Check sheet for the drawn part. Datum: minimum x, y, z corner. Units: mm. A direction names the side the tool comes from. Coordinates: 2 decimals unless noted, no trailing zeros. Write each loop counter-clockwise with the first axis right and the second up, starting at its lowest first coordinate (ties: lowest second). Pieces come first, ordered by that corner, then holes. Notation, with made-up numbers: M 69,-35.5 L 127,-35.5 A16 cw 127,-28.5 Z; hole C 67.5,0.5 d4. An arc over 180 degrees is marked long. Answer as CSV lines item,"result". Start each with the question number.
Q1. Mould release check, pull along X, two halves, no side actions. Record for the marked faces 1, 2, 3 and 4: pulls with the +X half, pulls with the -X half, needs draft (parallel to the pull), parting line crosses it, or undercut.
Q2. Thickness scan on line 1 along X through (y, z) = (13.5, 0.8); line 2 along Y through (x, z) = (22.5, 2.15). Record the ranges inside material, lowest first. Write a range as from..to.
Q3. Sectioned sample at A-A, the plane x = 13.5. Record the cut outline in (y, z).
Q4. Depth check by flat-ended pin: pin 1 Ø1.5 at (y, z) = (7.5, 2) entering from -X; pin 2 Ø1.5 at (x, z) = (6, 2) entering from -Y; pin 3 Ø1.5 at (x, z) = (21, 1.5) entering from +Y; pin 4 Ø3.5 at (x, y) = (22.5, 13.5) entering from -Z. Enter the tip coordinate at first touch or a pass-through.
Q5. Sectioned sample at D-D, the plane y = 21.5. Record the cut outline in (x, z), then the cut area to 3 significant figures.
Q6. Access from +Z, -Z, +X, -X, +Y, -Y to the whole of each face (thin tool, end or side, straight path). Record for the marked faces 5, 6, 7, 8 and 9.
Q7. Sectioned sample at C-C, the plane z = 1.35. Record the cut outline in (x, y).
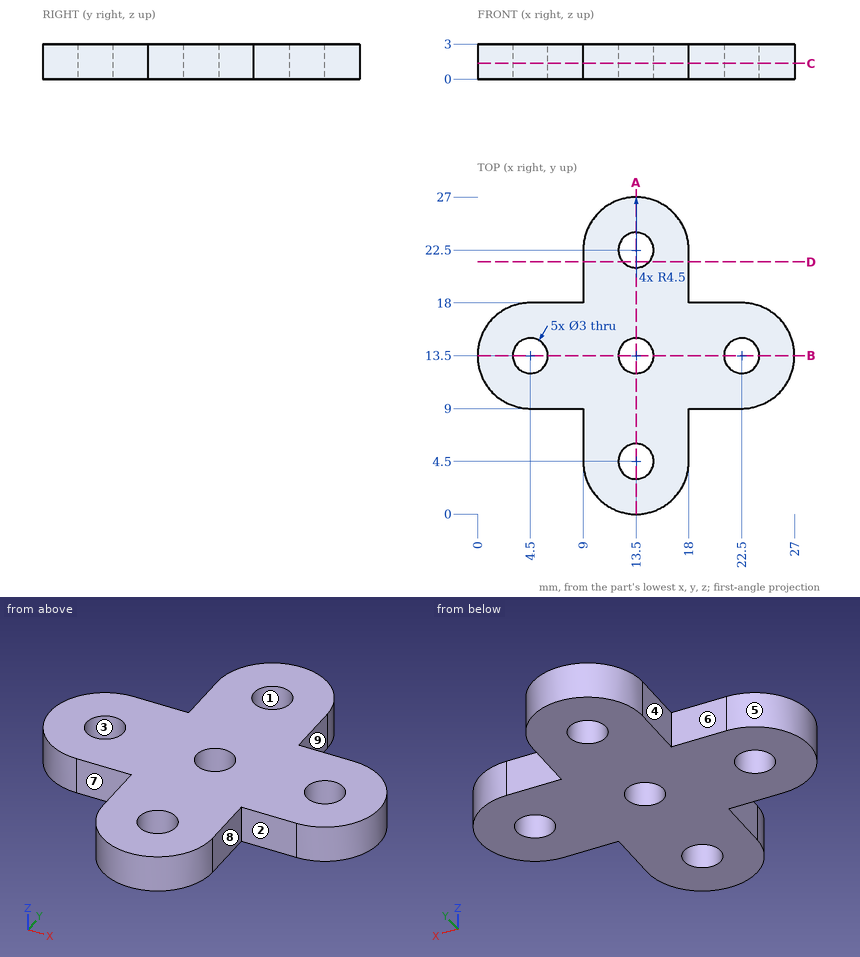
Output:
1,face 1,"undercut"
1,face 2,"needs draft"
1,face 3,"undercut"
1,face 4,"pulls with the -X half"
2,line 1,"x = 0..3, 6..12, 15..21, 24..27"
2,line 2,"y = 9..12, 15..18"
3,outline,"M 0,0 L 3,0 L 3,3 L 0,3 Z; M 6,0 L 12,0 L 12,3 L 6,3 Z; M 15,0 L 21,0 L 21,3 L 15,3 Z; M 24,0 L 27,0 L 27,3 L 24,3 Z"
4,pin 1,"stops at x = 9"
4,pin 2,"stops at y = 9"
4,pin 3,"stops at y = 18"
4,pin 4,"stops at z = 0"
5,outline,"M 9,0 L 12.38,0 L 12.38,3 L 9,3 Z; M 14.62,0 L 18,0 L 18,3 L 14.62,3 Z"
5,area,"20.3 mm^2"
6,face 5,"+Z, -Z, -X"
6,face 6,"+Z, -Z, -X, +Y"
6,face 7,"+Z, -Z, -X, -Y"
6,face 8,"+Z, -Z, +X, -Y"
6,face 9,"+Z, -Z, +X, +Y"
7,outline,"M 4.5,9 L 9,9 L 9,4.5 A4.5 ccw 18,4.5 L 18,9 L 22.5,9 A4.5 ccw 22.5,18 L 18,18 L 18,22.5 A4.5 ccw 9,22.5 L 9,18 L 4.5,18 A4.5 ccw Z; hole C 4.5,13.5 d3; hole C 13.5,4.5 d3; hole C 13.5,13.5 d3; hole C 13.5,22.5 d3; hole C 22.5,13.5 d3"
